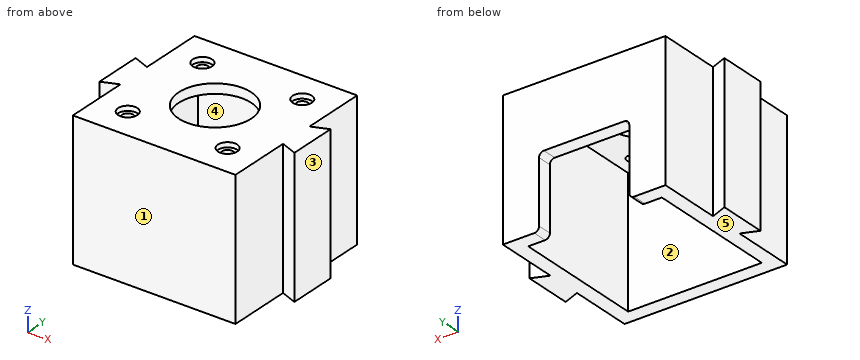
```python
from build123d import *

# Parameters (mm, degrees)
SKETCH1_W           = 50.5
SKETCH1_H           = 50.5
SKETCH1_R           = 11.25
SKETCH1_R_2         = 1.75
BOSS_EXTRUDE1_DEPTH = 3
SKETCH1_4_W         = 50.5
SKETCH1_4_H         = 50.5
SKETCH1_4_W_2       = 42.5
SKETCH1_4_H_2       = 42.5
BOSS_EXTRUDE2_DEPTH = 39.5
SKETCH6_W           = 42.5
SKETCH6_H           = 42.5
SKETCH6_W_2         = 41.5
SKETCH6_H_2         = 41.5
BOSS_EXTRUDE4_DEPTH = 39.5
CUT_EXTRUDE1_DEPTH  = 20
FILLET1_R           = 1.5
SKETCH4_R           = 3
CUT_EXTRUDE2_DEPTH  = 1.5
BOSS_EXTRUDE3_DEPTH = 42.5


with BuildPart() as part:
    # Sketch1 → Boss-Extrude1 (new body)
    with BuildSketch(Plane.XY):
        Rectangle(SKETCH1_W, SKETCH1_H)
        Circle(SKETCH1_R, mode=Mode.SUBTRACT)
        with Locations((-15.5, 15.5)):
            Circle(SKETCH1_R_2, mode=Mode.SUBTRACT)
        with Locations((15.5, 15.5)):
            Circle(SKETCH1_R_2, mode=Mode.SUBTRACT)
        with Locations((-15.5, -15.5)):
            Circle(SKETCH1_R_2, mode=Mode.SUBTRACT)
        with Locations((15.5, -15.5)):
            Circle(SKETCH1_R_2, mode=Mode.SUBTRACT)
    extrude(amount=BOSS_EXTRUDE1_DEPTH)

    # Sketch1<4> → Boss-Extrude2 (add)
    with BuildSketch(Plane.XY):
        Rectangle(SKETCH1_4_W, SKETCH1_4_H)
        Rectangle(SKETCH1_4_W_2, SKETCH1_4_H_2, mode=Mode.SUBTRACT)
    extrude(amount=-BOSS_EXTRUDE2_DEPTH)

    # Sketch6 → Boss-Extrude4 (add)
    with BuildSketch(Plane(origin=(0, 0, 0), x_dir=(-1, 0, 0), z_dir=(0, 0, -1))):
        Rectangle(SKETCH6_W, SKETCH6_H)
        Rectangle(SKETCH6_W_2, SKETCH6_H_2, mode=Mode.SUBTRACT)
    extrude(amount=BOSS_EXTRUDE4_DEPTH)

    # Sketch2 → Cut-Extrude1 (cut)
    with BuildSketch(Plane(origin=(0, 25.25, 0), x_dir=(1, 0, 0), z_dir=(0, 1, 0))):
        with BuildLine():
            Line((-14, 39.5), (14, 39.5))
            Line((14, 39.5), (14, 18.5))
            ThreePointArc((14, 18.5), (13.560660172, 17.439339828), (12.5, 17))
            Line((12.5, 17), (-12.5, 17))
            ThreePointArc((-12.5, 17), (-13.560660172, 17.439339828), (-14, 18.5))
            Line((-14, 18.5), (-14, 39.5))
        make_face()
    extrude(amount=-CUT_EXTRUDE1_DEPTH, mode=Mode.SUBTRACT)

    # Fillet1
    fillet1_edges = [part.edges().sort_by_distance(p)[0] for p in [
        (-14, 23, -39.5),
        (14, 23, -39.5),
    ]]
    fillet(fillet1_edges, radius=FILLET1_R)

    # Sketch4 → Cut-Extrude2 (cut)
    with BuildSketch(Plane.XY.offset(3)):
        with Locations((15.5, 15.5)):
            Circle(SKETCH4_R)
        with Locations((15.5, -15.5)):
            Circle(SKETCH4_R)
        with Locations((-15.5, 15.5)):
            Circle(SKETCH4_R)
        with Locations((-15.5, -15.5)):
            Circle(SKETCH4_R)
    extrude(amount=-CUT_EXTRUDE2_DEPTH, mode=Mode.SUBTRACT)

    # Sketch5 → Boss-Extrude3 (add)
    with BuildSketch(Plane.XY.offset(3)):
        Polygon((25.25, 5.5), (30.25, 7.5), (30.25, -7.5), (25.25, -5.5), align=None)
        Polygon((-30.25, -7.5), (-25.25, -5.5), (-25.25, 5.5), (-30.25, 7.5), align=None)
    extrude(amount=-BOSS_EXTRUDE3_DEPTH)


solid = part.part
```
CAD build for the part. Positions are in the model's coordinates, mm. Face numbers are marked on the shaded views. A direction names the side the tool comes from. Coordinates: 2 decimals unless noted, no trailing zeros. Loops run counter-clockwise (first coordinate to the right, second up) from the corner with the lowest first, then second, coordinate; pieces in that order, holes last. Notation, with made-up numbers: (51.25, -31) - (92.25, -31) arc R27 ccw to (92.25, -6) - close; hole circle Ø6 at (46.5, -25). An arc over 180 degrees is marked (long way). Return JSON: item names as keys, results as strings.
1. Band-saw the part on B-B (x = 0). Give the cut face in (y, z).
Result:
{"outline": "(-25.25, -39.5) - (-20.75, -39.5) - (-20.75, 0) - (-11.25, 0) - (-11.25, 3) - (-25.25, 3) - close; (11.25, 0) - (20.75, 0) - (20.75, -17) - (25.25, -17) - (25.25, 3) - (11.25, 3) - close"}
2. Band-saw the part on C-C (z = -6). Give the cut face in (x, y).
Result:
{"outline": "(-30.25, -7.5) - (-25.25, -5.5) - (-25.25, -25.25) - (25.25, -25.25) - (25.25, -5.5) - (30.25, -7.5) - (30.25, 7.5) - (25.25, 5.5) - (25.25, 25.25) - (-25.25, 25.25) - (-25.25, 5.5) - (-30.25, 7.5) - close; hole (-20.75, -20.75) - (20.75, -20.75) - (20.75, 20.75) - (-20.75, 20.75) - close"}
3. Drop flat-ended pins along their axis: pin 1 (10 mm diameter, centred on y = 15, z = -26.5, fed in from +X); pin 2 (3 mm diameter, centred on x = 14.5, y = -16.5, fed in from +Z); pin 3 (2 mm diameter, centred on x = -1.5, z = -29.5, fed in from +Y); pin 4 (3 mm diameter, centred on x = 15.5, y = -15.5, fed in from -Z). Give the stop position or say it passes through.
Result:
{"pin 1": "stops at x = 25.25", "pin 2": "stops at z = 1.5", "pin 3": "stops at y = -20.75", "pin 4": "passes through"}
4. Band-saw the part on D-D (y = 0). Give the cut face in (x, z).
Result:
{"outline": "(-30.25, -39.5) - (-20.75, -39.5) - (-20.75, 0) - (-11.25, 0) - (-11.25, 3) - (-30.25, 3) - close; (11.25, 0) - (20.75, 0) - (20.75, -39.5) - (30.25, -39.5) - (30.25, 3) - (11.25, 3) - close"}
5. Mould opens along X. For the marked faces 3, 4 and 5 say: released by +X, released by -X, zero draft, split by the parting line, or undercut.
Result:
{"face 3": "released by +X", "face 4": "undercut", "face 5": "zero draft"}
6. Band-saw the part on A-A (y = 15.5). Give the cut face in (x, z).
Result:
{"outline": "(-25.25, -39.5) - (-20.75, -39.5) - (-20.75, 0) - (-17.25, 0) - (-17.25, 1.5) - (-18.5, 1.5) - (-18.5, 3) - (-25.25, 3) - close; (-13.75, 0) - (13.75, 0) - (13.75, 1.5) - (12.5, 1.5) - (12.5, 3) - (-12.5, 3) - (-12.5, 1.5) - (-13.75, 1.5) - close; (17.25, 0) - (20.75, 0) - (20.75, -39.5) - (25.25, -39.5) - (25.25, 3) - (18.5, 3) - (18.5, 1.5) - (17.25, 1.5) - close"}
7. 3-axis set-ups, long thin cutter, end or side, ignore diameter. For the marked faces 1 and 2: which of +Z, -Z, +X, -X, +Y, -Y reach the whole face in a straight line?
Result:
{"face 1": "+Z, -Z, +X, -X, -Y", "face 2": "-Z"}
8. Probe L1, parallel to X at y = 15.5, z = 0.6; L2, parallel to Y at x = 15.5, z = 1.95. List the from-to ranges inside material, lowest first. Write a range as from..to.
Result:
{"L1": "x = -25.25..-17.25, -13.75..13.75, 17.25..25.25", "L2": "y = -25.25..-18.5, -12.5..12.5, 18.5..25.25"}
